For this review, take the finished solid that the model builds, in its own axes (mm). A direction names the side the tool comes from. Coordinates: 2 decimals unless noted, no trailing zeros. Write each loop counter-clockwise with the first axis right and the second up, starting at its lowest first coordinate (ties: lowest second). Pieces come first, ordered by that corner, then holes. Notation, with made-up numbers: (2, 32.25) -> (48, 32.25) arc R15 ccw to (48, 37.25) -> close; hole circle Ø8 at (43, 78). An arc over 180 degrees is marked (long way). Put each result on its own line as item: value. Start each with the question number.
Item 1: Consider section B-B on z = 9. Give the boundary of the cut face in (x, y), and give its area (3 significant figures).
Item 2: Insertion check: P1, Ø12, axis at x = 49.5, y = 39, coming from the -Z side; P2, Ø3, axis at x = 79.5, y = 44.5, coming from the +Z side; P3, Ø11, axis at x = 42.5, y = 3.5, coming from the +Z side. Each pin has a flat end and moves straight along its axis. Give the tip position at first contact, or say it passes through.
Item 3: To check wall thickness, follow L1, parallel to Y at x = 26, z = -12; L2, parallel to Z at x = 44, y = 12; L3, parallel to Y at x = 90, z = 27. State the ranges of each line that lie inside material, in increasing order.
Item 4: For faces 1 (the cylindrical face through (89.15, 43.92, 44.43)), 2 (the flat face through (47, 8, 13.449)), 3 (the flat face through (47, 18.596, -7)), 4 (the flat face through (50, 92.596, 56)), list the 3-axis set-ups (+Z, -Z, +X, -X, +Y, -Y) from which the entire face can be reached by the end or side of a thin tool; tool diameter is ignored.
Item 5: Consider section C-C on y = 14. Give the boundary of the cut face in (x, z), and give its area (3 significant figures).
Item 6: Consider section A-A on x = 51. Give the boundary of the cut face in (y, z).
Item 7: Consider section D-D on y = 57.5. Give the boundary of the cut face in (x, z).
```python
from build123d import *

# Parameters (mm, degrees)
BOSS_EXTRUDE1_DEPTH = 96
SKETCH2_R           = 40
BOSS_EXTRUDE2_DEPTH = 96


with BuildPart() as part:
    # Sketch1 → Boss-Extrude1 (new body)
    with BuildSketch(Plane(origin=(0, 0, 0), x_dir=(0, 0, -1), z_dir=(1, 0, 0))):
        Polygon((-101.449299301, -56.403624436), (26.550700699, -56.403624436), (26.550700699, -3.403624436), (26.550700699, 18.596375564), (-13.449299301, 18.596375564), (-13.449299301, -3.403624436), (-101.449299301, -3.403624436), align=None)
    extrude(amount=BOSS_EXTRUDE1_DEPTH)

    # Sketch2 → Boss-Extrude2 (add)
    with BuildSketch(Plane(origin=(0, -3.403624436, 0), x_dir=(1, 0, 0), z_dir=(0, 1, 0))):
        with Locations((51, -56.449299301)):
            Circle(SKETCH2_R)
    extrude(amount=BOSS_EXTRUDE2_DEPTH)


solid = part.part
```
Return value:
1. outline: (0, -56.4) -> (96, -56.4) -> (96, 18.6) -> (0, 18.6) -> close
1. area: 7,200 mm^2
2. P1: z = 16.45
2. P2: z = 85.96
2. P3: z = 96.34
3. L1: -56.4 to 18.6
3. L2: -26.55 to 13.45, 17.07 to 95.83
3. L3: -56.4 to -3.4
4. face 1: +Y
4. face 2: +X, -X, +Y
4. face 3: -Z, +X, -X, +Y
4. face 4: +Z, -Z, +X, -X, +Y
5. outline: (0, -26.55) -> (96, -26.55) -> (96, 13.45) -> (0, 13.45) -> close; circle Ø80 at (51, 56.45)
5. area: 8,870 mm^2
6. outline: (-56.4, -26.55) -> (18.6, -26.55) -> (18.6, 13.45) -> (-3.4, 13.45) -> (-3.4, 16.45) -> (92.6, 16.45) -> (92.6, 96.45) -> (-3.4, 96.45) -> (-3.4, 101.45) -> (-56.4, 101.45) -> close
7. outline: circle Ø80 at (51, 56.45)
